Can you work these out from the model? Positions are in its coordinate system, mm. A direction names the side the tool comes from. Coordinates: 2 decimals unless noted, no trailing zeros. Order: outer loops, then holes, each group sorted by start corner. A loop starts at its lowest first (then second) coordinate and runs counter-clockwise, first axis right, second up. Notation, with made-up numbers: (82.5, -18.75) -> (140.5, -18.75) arc R17 cw to (140.5, 14.25) -> close; hole circle Ø9 at (33.25, 78.5). An arc over 180 degrees is marked (long way). Return JSON: item names as keys, results as strings. Group by question number.
1) If we section it at B-B, the plane z = 15: State how many separate pieces and enclosed holes the cut face has, then the cut area to 3 significant figures.
2) Thinking about a two-plate mould opening in X: for faces 1 (the flat face through (8.2, -12.4, 0)), 2 (the flat face through (19.05, 0, 13)), 3 (the cylindrical face through (11.85, 14.18, 12.52)), which applies, +X half, -X half, draft (parallel to the pull), parting line (faces both ways), or undercut?
3) For pin 1 (16 mm diameter, centred on x = -1, y = -5, fed in from -Z); pin 2 (16 mm diameter, centred on x = -5.5, y = 6, fed in from +Z), each with a flat end and sliding along its axis, tell me the tip position at first contact or that it passes through.
4) For faces 4 (the cylindrical face through (15.14, 6.36, 24.62)), 5 (the flat face through (13, 8, 1.588)), 6 (the flat face through (0, -19.05, 13)), which set-ups out of +Z, -Z, +X, -X, +Y, -Y let a thin tool reach every point of the face, with its end or its side?
5) If I drill on probe 1 along X at (y, z) = (-14.5, 10); probe 2 along X at (y, z) = (14.5, 3); probe 3 along Y at (x, z) = (15.5, 7), over which ranges is the centre line in solid material (lowest first)? Write a range as from..to.
6) If we section it at C-C, the plane y = -2: Please give me the cut outline in (x, z).
7) If we section it at D-D, the plane y = -15: Please give me the cut outline in (x, z), then the cut area to 3 significant figures.
Autodesk Inventor part; units mm, degrees
ref_plane "YZ Plane" through (0, 0, 0) normal (1, 0, 0) x (0, 1, 0)
ref_plane "XZ Plane" through (0, 0, 0) normal (0, 1, 0) x (-1, 0, 0)
ref_plane "XY Plane" through (0, 0, 0) normal (0, 0, 1) x (1, 0, 0)
sketch "Sketch1" plane through (0, 0, 0) normal (0, 0, 1) x (1, 0, 0)
  line L0 (-19.05, 19.05) -> (19.05, 19.05)
  line L1 (19.05, 19.05) -> (19.05, -19.05)
  line L2 (19.05, -19.05) -> (-19.05, -19.05)
  line L3 (-19.05, -19.05) -> (-19.05, 19.05)
  circle A0 centre (-14.2875, 14.2875) radius 2.4384
  circle A1 centre (14.2875, 14.2875) radius 2.4384
  circle A2 centre (14.2875, -14.2875) radius 2.4384
  circle A3 centre (-14.2875, -14.2875) radius 2.4384
  line L4 (-19.05, 15.875) -> (19.05, 15.875) construction
  line L5 (14.2875, 19.05) -> (14.2875, -19.05) construction
  line L6 (19.05, -12.7) -> (-19.05, -12.7) construction
  line L7 (-14.2875, -19.05) -> (-14.2875, 19.05) construction
  circle A4 centre (0, 1.5875) radius 14.2875
  point P0 (0, 0)
  dimension "d2" = 38.1
  dimension "d4" = 38.1
  dimension "d5" = 4.8768
  dimension "d6" = 4.7625
  dimension "d7" = 4.7625
  dimension "d8" = 4.7625
  dimension "d9" = 4.7625
  dimension "d10" = 4.7625
  dimension "d11" = 4.7625
  dimension "d12" = 4.7625
  dimension "d13" = 4.7625
  dimension "d22" = 19.05
  dimension "d23" = 6.35
extrude "Extrusion4" add sketch "Sketch1" along normal blind 25.4
sketch "Sketch4" plane through (0, 0, 25.4) normal (0, 0, 1) x (1, 0, 0)
  circle A0 centre (0, 1.5875) radius 14.2875
  circle A1 centre (0, 1.5875) radius 15.875
  circle A2 centre (0, 1.5875) radius 14.2875
  point P0 (0, 0)
  dimension "d26" = 1.5875
extrude "Extrusion5" cut sketch "Sketch4" against normal blind 1.5875
sketch "Sketch5" plane through (0, 0, 0) normal (0, 0, -1) x (-1, 0, 0)
  circle A0 centre (0, 1.5875) radius 14.2875
  circle A1 centre (0, 1.5875) radius 15.875
  circle A2 centre (0, 1.5875) radius 14.2875
  point P0 (0, 0)
  dimension "d29" = 1.5875
extrude "Extrusion6" cut sketch "Sketch5" against normal blind 1.5875
properties part number "WheelBearingBlock" material "Aluminum-6061"
Result sheet:
{
 "1": {"separate pieces": "1", "enclosed holes": "5", "area": "736 mm2"},
 "2": {"face 1": "draft", "face 2": "+X half", "face 3": "undercut"},
 "3": {"pin 1": "stops at z = 1.59", "pin 2": "stops at z = 23.81"},
 "4": {"face 4": "+Z", "face 5": "-Z", "face 6": "+Z, -Z, +X, -X, -Y"},
 "5": {"probe 1": "x = -19.05..-16.72, -11.86..11.86, 16.72..19.05", "probe 2": "x = -19.05..-16.72, -11.86..-6.12, 6.12..11.86, 16.72..19.05", "probe 3": "y = -19.05..-16.4, -12.17..12.17, 16.4..19.05"},
 "6": {"outline": "(-19.05, 0) -> (-15.46, 0) -> (-15.46, 1.59) -> (-13.83, 1.59) -> (-13.83, 23.81) -> (-15.46, 23.81) -> (-15.46, 25.4) -> (-19.05, 25.4) -> close; (13.83, 1.59) -> (15.46, 1.59) -> (15.46, 0) -> (19.05, 0) -> (19.05, 25.4) -> (15.46, 25.4) -> (15.46, 23.81) -> (13.83, 23.81) -> close"},
 "7": {"outline": "(-19.05, 0) -> (-16.62, 0) -> (-16.62, 25.4) -> (-19.05, 25.4) -> close; (-11.96, 0) -> (11.96, 0) -> (11.96, 25.4) -> (-11.96, 25.4) -> close; (16.62, 0) -> (19.05, 0) -> (19.05, 25.4) -> (16.62, 25.4) -> close", "area": "731 mm2"}
}
